```python
from build123d import *

# Parameters (mm, degrees)
CROQUIS1_W              = 485
CROQUIS1_H              = 89
SALIENTE_EXTRUIR1_DEPTH = 16
CORTAR_EXTRUIR2_DEPTH   = 89
CORTAR_EXTRUIR3_DEPTH   = 89
CORTAR_EXTRUIR4_DEPTH   = 89


with BuildPart() as part:
    # Croquis1 → Saliente-Extruir1 (new body)
    with BuildSketch(Plane(origin=(0, 0, 0), x_dir=(1, 0, 0), z_dir=(0, 1, 0))):
        Rectangle(CROQUIS1_W, CROQUIS1_H)
    extrude(amount=SALIENTE_EXTRUIR1_DEPTH)

    # Croquis2 → Cortar-Extruir2 (cut)
    with BuildSketch(Plane.XY.offset(44.5)):
        with BuildLine():
            ThreePointArc((-234.5, 0), (-240.156854249, 2.343145751), (-242.5, 8))
            Line((-242.5, 8), (-242.5, 0))
            Line((-242.5, 0), (-234.5, 0))
        make_face()
        with BuildLine():
            ThreePointArc((-242.5, 8), (-240.156854236, 13.656854263), (-234.499999961, 16))
            Line((-234.499999961, 16), (-242.5, 16))
            Line((-242.5, 16), (-242.5, 8))
        make_face()
    extrude(amount=-CORTAR_EXTRUIR2_DEPTH, mode=Mode.SUBTRACT)

    # Croquis3 → Cortar-Extruir3 (cut)
    with BuildSketch(Plane.XY.offset(44.5)):
        with BuildLine():
            Line((242.5, 16), (234.5, 16))
            ThreePointArc((234.5, 16), (240.156854249, 13.656854249), (242.5, 8))
            Line((242.5, 8), (242.5, 16))
        make_face()
        with BuildLine():
            Line((242.5, 0), (242.5, 8))
            ThreePointArc((242.5, 8), (240.156854249, 2.343145751), (234.5, 0))
            Line((234.5, 0), (242.5, 0))
        make_face()
    extrude(amount=-CORTAR_EXTRUIR3_DEPTH, mode=Mode.SUBTRACT)

    # Croquis4 → Cortar-Extruir4 (cut)
    with BuildSketch(Plane.XY.offset(44.5)):
        with BuildLine():
            Line((-234.5, 15.5), (234.5, 15.5))
            ThreePointArc((234.5, 15.5), (242, 8), (234.5, 0.5))
            Line((234.5, 0.5), (-234.5, 0.5))
            ThreePointArc((-234.5, 0.5), (-242, 8), (-234.5, 15.5))
        make_face()
    extrude(amount=-CORTAR_EXTRUIR4_DEPTH, mode=Mode.SUBTRACT)


solid = part.part
```
CAD build for the part. Positions are in the model's coordinates, mm. A direction names the side the tool comes from. Round coordinates to 2 decimals unless told otherwise and drop trailing zeros. Order: outer loops, then holes, each group sorted by start corner. A loop starts at its lowest first (then second) coordinate and runs counter-clockwise, first axis right, second up. Notation, with made-up numbers: (86, 41.5) - (96, 41.5) arc R19 ccw to (96, 68.5) - close; hole circle Ø9 at (-18, 26.5). An arc over 180 degrees is marked (long way). Answer as CSV lines item,"result". Start each with the question number.
1. Saw through at C-C, the plane y = 12. Write the cut outline in (x, z), and give its area (3 significant figures).
2. Saw through at A-A, the plane x = 209. Write the cut outline in (y, z), and give its area (3 significant figures).
3. Drill centre lines: L1, parallel to Y at x = 197, z = 38; L2, parallel to X at y = 7.5, z = -29.5; L3, parallel to X at y = 10.5, z = -22. Where is each one in solid material? Low to high. Write a range as [from, to].
4. Tool access for faces 1 (the face through (-3, 15.5, 1)), 2 (the face through (-1.1, 15.7, 44.5)): list every direction of +Z, -Z, +X, -X, +Y, -Y with a clear straight run to the whole face (end or side of a thin tool).
5. Pull direction X, two halves, no side cores. Call faces 3 (the face through (3, 0.5, 1)), 4 (the face through (-3, 16, -1)): +X half, -X half, draft (parallel to the pull), parting line (faces both ways), or undercut.
6. Saw through at B-B, the plane z = -2. Write the cut outline in (x, y), and give its area (3 significant figures).
7. Pin check, flat tip, straight feed: pin 1 (1 mm diameter, centred on y = 4, z = -26.5, fed in from -X). Stop position of the tip, or through.
Model answer:
1,outline,"(-241.43, -44.5) - (-240.84, -44.5) - (-240.84, 44.5) - (-241.43, 44.5) - close; (240.84, -44.5) - (241.43, -44.5) - (241.43, 44.5) - (240.84, 44.5) - close"
1,area,"104 mm²"
2,outline,"(0, -44.5) - (0.5, -44.5) - (0.5, 44.5) - (0, 44.5) - close; (15.5, -44.5) - (16, -44.5) - (16, 44.5) - (15.5, 44.5) - close"
2,area,"89.0 mm²"
3,L1,"y = [0, 0.5], [15.5, 16]"
3,L2,"x = [-242.48, -241.98], [241.98, 242.48]"
3,L3,"x = [-242.1, -241.57], [241.57, 242.1]"
4,face 1,"+Z, -Z"
4,face 2,"+Z, +X, -X, +Y, -Y"
5,face 3,"undercut"
5,face 4,"draft"
6,outline,"(-234.5, 0) - (234.5, 0) arc R8 ccw to (234.5, 16) - (-234.5, 16) arc R8 ccw to start; hole (-234.5, 0.5) - (234.5, 0.5) arc R7.5 ccw to (234.5, 15.5) - (-234.5, 15.5) arc R7.5 ccw to start"
6,area,"493 mm²"
7,pin 1,"stops at x = -241.69"
